Can you work these out from the model? Positions are in its coordinate system, mm. Face numbers are marked on the shaded views. A direction names the side the tool comes from. Coordinates: 2 decimals unless noted, no trailing zeros. Order: outer loops, then holes, each group sorted by start corner. A loop starts at its lowest first (then second) coordinate and runs counter-clockwise, first axis right, second up. Notation, with made-up numbers: M -27.75,25 L -20.75,25 A21 cw -20.75,54 Z; hole C 8.5,-37.75 d8. An arc over 180 degrees is marked long. Answer as a JSON object with one key per item and string values.
from build123d import *

# Parameters (mm, degrees)
F0_W     = 49.022
F0_H     = 107.95
F1_DEPTH = 12.7
F2_R     = 5.715
F3_DEPTH = 2.54
F4_W     = 37.592
F4_H     = 96.52
F5_DEPTH = 1.905
F6_W     = 53.975
F6_H     = 9.398
F7_DEPTH = 15.875
F8_W     = 53.975
F8_H     = 9.398
F9_DEPTH = 15.875


with BuildPart() as f1:
    # F0 (on Top) → F1 (new body)
    with BuildSketch(Plane.XY):
        Rectangle(F0_W, F0_H)
    extrude(amount=F1_DEPTH)

    # F2 (on face) → F3 (cut)
    with BuildSketch(Plane(origin=(0, 0, 0), x_dir=(1, 0, 0), z_dir=(0, 0, -1))):
        Circle(F2_R)
    extrude(amount=-F3_DEPTH, mode=Mode.SUBTRACT)

    # F4 (on face) → F5 (cut)
    with BuildSketch(Plane.XY.offset(12.7)):
        Rectangle(F4_W, F4_H)
    extrude(amount=-F5_DEPTH, mode=Mode.SUBTRACT)

    # F6 (on face) → F7 (cut)
    with BuildSketch(Plane(origin=(-24.511, 0, 0), x_dir=(0, -1, 0), z_dir=(-1, 0, 0))):
        with Locations((0, 5.969)):
            Rectangle(F6_W, F6_H)
    extrude(amount=-F7_DEPTH, mode=Mode.SUBTRACT)

    # F8 (on face) → F9 (cut)
    with BuildSketch(Plane.YZ.offset(24.511)):
        with Locations((0, 5.969)):
            Rectangle(F8_W, F8_H)
    extrude(amount=-F9_DEPTH, mode=Mode.SUBTRACT)


solid = f1.part
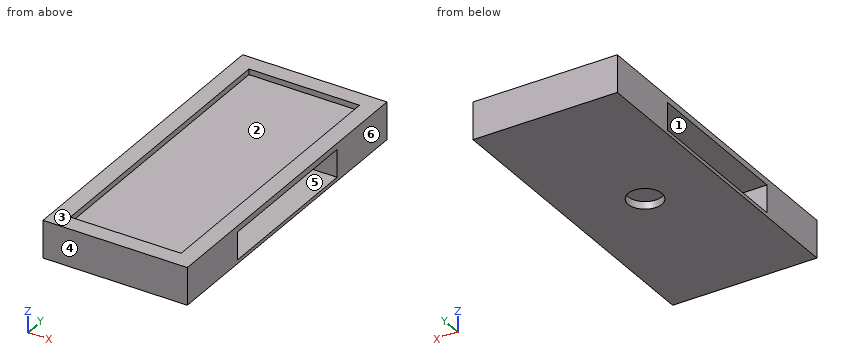
Item 1: I want a section at B-B, the plane z = 8.25. Write out the boundary of the cut face in (x, y) (1 decimal), plus the area to 3 significant figures.
Answers follow:
{"outline": "M -24.5,-54 L 24.5,-54 L 24.5,-27 L 8.6,-27 L 8.6,27 L 24.5,27 L 24.5,54 L -24.5,54 L -24.5,27 L -8.6,27 L -8.6,-27 L -24.5,-27 Z", "area": "3,580 mm^2"}
Item 2: If we mould it in two halves opening along Y, with no side actions, what happens to the marked faces 1, 2, 3 and 4? For each: pulls with the +Y half, pulls with the -Y half, needs draft (parallel to the pull), parting line crosses it, or undercut.
Answers follow:
{"face 1": "undercut", "face 2": "undercut", "face 3": "needs draft", "face 4": "pulls with the -Y half"}
Item 3: Please list where these lines run through material, in increasing order: line 1 (X direction, y = 0, z = 1.15) (3 decimals); line 2 (Y direction, x = -9, z = 4.5) (1 decimal); line 3 (Y direction, x = 0, z = 1.1) (3 decimals).
Answers follow:
{"line 1": "x = -24.511 to -5.715, 5.715 to 24.511", "line 2": "y = -54 to -27, 27 to 54", "line 3": "y = -53.975 to -5.715, 5.715 to 53.975"}
Item 4: I'm going to push flat-ended pins straight in: pin 1 (7 mm diameter, centred on x = 0, y = 0, fed in from +Z) (3 decimals); pin 2 (2 mm diameter, centred on y = -5.5, z = 3.5, fed in from -X); pin 3 (1 mm diameter, centred on y = 10, z = 5, fed in from +X). Where does each tip first touch, or does it pass through?
Answers follow:
{"pin 1": "stops at z = 10.795", "pin 2": "stops at x = -8.64", "pin 3": "stops at x = 8.64"}
Item 5: I want a section at C-C, the plane x = 15. Write out the boundary of the cut face in (y, z) (1 decimal), plus the area to 3 significant figures.
Answers follow:
{"outline": "M -54,0 L 54,0 L 54,12.7 L 48.3,12.7 L 48.3,10.8 L -48.3,10.8 L -48.3,12.7 L -54,12.7 Z; hole M -27,1.3 L 27,1.3 L 27,10.7 L -27,10.7 Z", "area": "680 mm^2"}
Item 6: I want a section at A-A, the plane y = 0. Write out the boundary of the cut face in (x, z) (3 decimals), plus the area to 3 significant figures.
Answers follow:
{"outline": "M -24.511,0 L -5.715,0 L -5.715,2.54 L 5.715,2.54 L 5.715,0 L 24.511,0 L 24.511,1.27 L 8.636,1.27 L 8.636,10.668 L 24.511,10.668 L 24.511,12.7 L 18.796,12.7 L 18.796,10.795 L -18.796,10.795 L -18.796,12.7 L -24.511,12.7 L -24.511,10.668 L -8.636,10.668 L -8.636,1.27 L -24.511,1.27 Z", "area": "224 mm^2"}
Item 7: Which directions (+Z, -Z, +X, -X, +Y, -Y) give clear straight access to the entire face, cutting with the end or side of a thin tool? Please do the marked faces 5 and 6.
Answers follow:
{"face 5": "+X", "face 6": "+Z, -Z, +X, +Y, -Y"}
Item 8: I want a section at D-D, the plane x = 0. Write out the boundary of the cut face in (y, z) (3 decimals), plus the area to 3 significant figures.
Answers follow:
{"outline": "M -53.975,0 L -5.715,0 L -5.715,2.54 L 5.715,2.54 L 5.715,0 L 53.975,0 L 53.975,12.7 L 48.26,12.7 L 48.26,10.795 L -48.26,10.795 L -48.26,12.7 L -53.975,12.7 Z", "area": "1,160 mm^2"}
